from build123d import *

# Parameters (mm, degrees)
F2_R     = 9.931182
F3_DEPTH = 50.8


with BuildPart() as f1:
    # F0 (on Front) → F1 (revolve)
    with BuildSketch(Plane.XZ):
        Polygon((0, -25.4), (0, 0), (54.017087, 53.745644), (51.690166, 55.812778), (-1.909546, 2.482411), (-12.7, 2.482411), (-12.7, -25.4), align=None)
    revolve(axis=Axis((-12.7, 0, -11.458795), (0, 0, 1)))

    # F2 (on face) → F3 (cut)
    with BuildSketch(Plane.XY.offset(2.482411)):
        with Locations((-12.7, 0)):
            Circle(F2_R)
    extrude(amount=-F3_DEPTH, mode=Mode.SUBTRACT)


solid = f1.part
Build history of the part. All positions in model axes, mm. A direction names the side the tool comes from. Coordinates: 2 decimals unless noted, no trailing zeros. Order: outer loops, then holes, each group sorted by start corner. A loop starts at its lowest first (then second) coordinate and runs counter-clockwise, first axis right, second up. Notation, with made-up numbers: (56.25, 70) - (115.25, 70) arc R19 ccw to (115.25, 84) - close; hole circle Ø1 at (68.5, 81). An arc over 180 degrees is marked (long way). Write each question's results on one line, items separated by ' | '. Start each with the question number.
Item 1: Wall check: probe 1 along Y at (x, z) = (-12, -16); probe 2 along X at (y, z) = (-2, -9.5); probe 3 along Y at (x, z) = (5.5, 42.5). Give the ranges that are in metal, low to high. Write a range as [from, to].
Item 2: Band-saw the part on B-B on y = 0. Write the cut outline in (x, z), and give its area (3 significant figures).
Item 3: Tool access for faces 1 (the face through (5.173, -7.411, 10.997)), 2 (the face through (-0.586, 3.815, -12.522)): list every direction of +Z, -Z, +X, -X, +Y, -Y with a clear straight run to the whole face (end or side of a thin tool).
Item 4: Flat gauge pins, fed straight in: pin 1 (2 mm diameter, centred on x = -18, z = 21.5, fed in from -Y); pin 2 (8 mm diameter, centred on y = -16, z = 24, fed in from -X); pin 3 (6 mm diameter, centred on x = -4.5, z = -3, fed in from +Y); pin 4 (16 mm diameter, centred on x = -12.7, y = 0, fed in from +Z). Where does each tip first touch, or does it go through?
Item 5: Band-saw the part on A-A on x = -12.7. Write the cut outline in (y, z), and give its area (3 significant figures).
Item 6: Band-saw the part on C-C on z = -4.5. Write the cut outline in (x, y), and give its area (3 significant figures).
Item 7: Mould opens along Y. For faces 3 (the face through (-5, -7, -25.4)), 4 (the face through (-63.89, -39.25, 55.71)), 5 (the face through (-8, -9, 2.482)) say: released by +Y, released by -Y, zero draft, split by the parting line, or undercut.
Item 8: Band-saw the part on D-D on z = 38.5. Write the cut outline in (x, y), and give its area (3 significant figures).
Numbers:
1) probe 1: [-12.68, -9.91], [9.91, 12.68] | probe 2: [-25.24, -22.43], [-2.97, -0.16] | probe 3: [-52.34, -47.65], [47.65, 52.34]
2) outline: (-79.42, 53.75) - (-25.4, 0) - (-25.4, -25.4) - (-22.63, -25.4) - (-22.63, 2.48) - (-23.49, 2.48) - (-77.09, 55.81) - close; (-2.77, -25.4) - (0, -25.4) - (0, 0) - (54.02, 53.75) - (51.69, 55.81) - (-1.91, 2.48) - (-2.77, 2.48) - close | area: 621 mm^2
3) face 1: +Z | face 2: -Z
4) pin 1: y = -34.92 | pin 2: x = -50.57 | pin 3: y = 11.59 | pin 4: through
5) outline: (-66.72, 53.75) - (-12.7, 0) - (-12.7, -25.4) - (-9.93, -25.4) - (-9.93, 2.48) - (-10.79, 2.48) - (-64.39, 55.81) - close; (9.93, -25.4) - (12.7, -25.4) - (12.7, 0) - (66.72, 53.75) - (64.39, 55.81) - (10.79, 2.48) - (9.93, 2.48) - close | area: 621 mm^2
6) outline: circle Ø25.4 at (-12.7, 0); hole circle Ø19.86 at (-12.7, 0) | area: 197 mm^2
7) face 3: zero draft | face 4: split by the parting line | face 5: undercut
8) outline: circle Ø102.79 at (-12.7, 0); hole circle Ø93.98 at (-12.7, 0) | area: 1,360 mm^2
